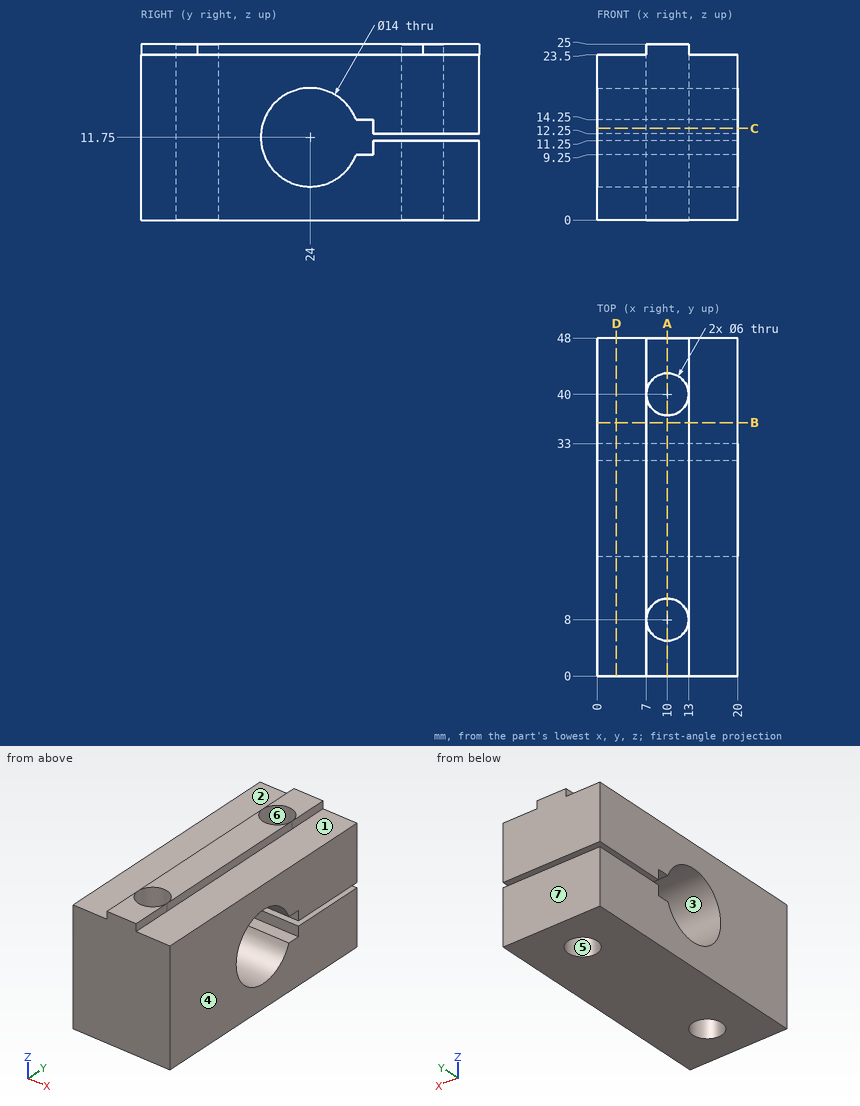
Verification items for this drawing (mm, ordinates from the low corner). A direction names the side the tool comes from. Coordinates: 2 decimals unless noted, no trailing zeros. Loops run counter-clockwise (first coordinate to the right, second up) from the corner with the lowest first, then second, coordinate; pieces in that order, holes last. Notation, with made-up numbers: (70, 36) - (81, 36) arc R17 ccw to (81, 46) - close; hole circle Ø8 at (0.5, 14.5). An arc over 180 degrees is marked (long way). Answer as a JSON object with one key per item and string values.
(1) Cross-section at C-C, the plane z = 13. Record the boundary of the cut face in (x, y).
Response:
{"outline": "(0, 0) - (20, 0) - (20, 17.11) - (0, 17.11) - close; (0, 33) - (20, 33) - (20, 48) - (0, 48) - close; hole circle Ø6 at (10, 8); hole circle Ø6 at (10, 40)"}
(2) Cross-section at D-D, the plane x = 2.75. Record the boundary of the cut face in (y, z).
Response:
{"outline": "(0, 0) - (48, 0) - (48, 11.25) - (33, 11.25) - (33, 9.25) - (30.54, 9.25) arc R7 cw (long way) to (30.54, 14.25) - (33, 14.25) - (33, 12.25) - (48, 12.25) - (48, 23.5) - (0, 23.5) - close"}
(3) Mould release check, pull along X, two halves, no side actions. Record for the marked faces 4, 5, 6 and 7: pulls with the +X half, pulls with the -X half, needs draft (parallel to the pull), parting line crosses it, or undercut.
Response:
{"face 4": "pulls with the +X half", "face 5": "undercut", "face 6": "undercut", "face 7": "needs draft"}
(4) Scan lines: line 1 along Y through (x, z) = (10, 21.5); line 2 along Z through (x, y) = (13.25, 44.5); line 3 along Y through (x, z) = (10, 14). Record each from-to range of solid material in increasing order.
Response:
{"line 1": "y = 0 to 5, 11 to 37, 43 to 48", "line 2": "z = 0 to 11.25, 12.25 to 23.5", "line 3": "y = 0 to 5, 11 to 17.37, 33 to 37, 43 to 48"}
(5) Go/stop test with flat-tipped pins: pin 1 Ø4 at (x, y) = (3, 13) entering from +Z; pin 2 Ø1.6 at (y, z) = (21.5, 24.5) entering from +X; pin 3 Ø4 at (x, y) = (10.5, 40.5) entering from -Z; pin 4 Ø0.8 at (y, z) = (16.5, 24) entering from -X. Record where each tip stops, or that it passes through.
Response:
{"pin 1": "stops at z = 23.5", "pin 2": "stops at x = 13", "pin 3": "passes through", "pin 4": "stops at x = 7"}
(6) Cross-section at B-B, the plane y = 36. Record the boundary of the cut face in (x, z).
Response:
{"outline": "(0, 0) - (20, 0) - (20, 11.25) - (0, 11.25) - close; (0, 12.25) - (20, 12.25) - (20, 23.5) - (13, 23.5) - (13, 25) - (7, 25) - (7, 23.5) - (0, 23.5) - close"}
(7) Access from +Z, -Z, +X, -X, +Y, -Y to the whole of each face (thin tool, end or side, straight path). Record for the marked faces 1, 2 and 3.
Response:
{"face 1": "+Z, +X, +Y, -Y", "face 2": "+Z, -X, +Y, -Y", "face 3": "+X, -X"}
(8) Cross-section at A-A, the plane x = 10. Record the boundary of the cut face in (y, z).
Response:
{"outline": "(0, 0) - (5, 0) - (5, 25) - (0, 25) - close; (11, 0) - (37, 0) - (37, 11.25) - (33, 11.25) - (33, 9.25) - (30.54, 9.25) arc R7 cw (long way) to (30.54, 14.25) - (33, 14.25) - (33, 12.25) - (37, 12.25) - (37, 25) - (11, 25) - close; (43, 0) - (48, 0) - (48, 11.25) - (43, 11.25) - close; (43, 12.25) - (48, 12.25) - (48, 25) - (43, 25) - close"}
